Part model, mm, in its own coordinate system. Face numbers are marked on the shaded views. A direction names the side the tool comes from. Round coordinates to 2 decimals unless told otherwise and drop trailing zeros. Write each loop counter-clockwise with the first axis right and the second up, starting at its lowest first coordinate (ties: lowest second). Pieces come first, ordered by that corner, then holes.
1) Saw through at C-C on x = 18.4. Write the cut outline in (y, z), and give its area (3 significant figures).
2) Drill centre lines: L1, parallel to X at y = -27.5, z = 1.15; L2, parallel to X at y = -23.25, z = 3.6; L3, parallel to Y at x = 18.4, z = 3.8. Where is each one in solid material? Low to high.
3) Which spindle directions (+Z, -Z, +X, -X, +Y, -Y) get a long thin tool onto all of the face, cutting with end or side? Do the marked faces 1, 2 and 3. Say none if no direction does.
4) Saw through at B-B on y = -25.75. Write the cut outline in (x, z), and give its area (3 significant figures).
5) Flat gauge pins, fed straight in: pin 1 (6 mm diameter, centred on x = 14.5, y = -29, fed in from -Z); pin 2 (1.5 mm diameter, centred on x = 22, z = 1.5, fed in from +Y). Where does each tip first touch, or does it go through?
6) Saw through at D-D on z = 5.1. Write the cut outline in (x, y), and give its area (3 significant figures).
7) Pull direction Y, two halves, no side cores. Call the marked faces 4, 5 and 6: +Y half, -Y half, draft (parallel to the pull), parting line (faces both ways), or undercut.
8) Saw through at A-A on z = 1.85. Write the cut outline in (x, y), and give its area (3 significant figures).
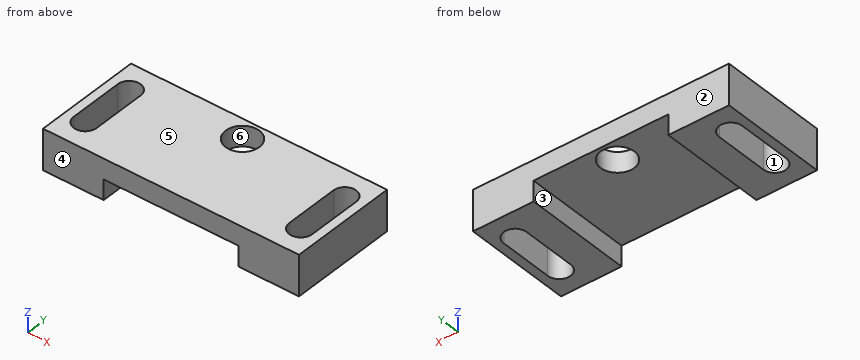
Autodesk Inventor part; units mm, degrees
ref_plane "YZ Plane" through (0, 0, 0) normal (1, 0, 0) x (0, 1, 0)
ref_plane "XZ Plane" through (0, 0, 0) normal (0, 1, 0) x (-1, 0, 0)
ref_plane "XY Plane" through (0, 0, 0) normal (0, 0, 1) x (1, 0, 0)
ref_plane "Work Plane1" through (0, 0, 0) normal (0, 0, 1) x (1, 0, 0)
sketch "Sketch1" plane through (0, 0, 0) normal (0, 0, 1) x (1, 0, 0)
  circle A0 centre (2.4, -23.5737) radius 1.4
  circle A1 centre (34.4, -23.5737) radius 1.4
  line L0 (2.4, -27.5737) -> (2.4, -19.5737) construction
  line L1 (4.1, -27.5737) -> (4.1, -19.5737)
  line L2 (0.7, -19.5737) -> (0.7, -27.5737)
  arc A2 (0.7, -27.5737) -> (4.1, -27.5737) centre (2.4, -27.5737) ccw
  arc A3 (4.1, -19.5737) -> (0.7, -19.5737) centre (2.4, -19.5737) ccw
  line L3 (34.4, -19.5737) -> (34.4, -27.5737) construction
  line L4 (32.7, -19.5737) -> (32.7, -27.5737)
  line L5 (36.1, -27.5737) -> (36.1, -19.5737)
  arc A4 (36.1, -19.5737) -> (32.7, -19.5737) centre (34.4, -19.5737) ccw
  arc A5 (32.7, -27.5737) -> (36.1, -27.5737) centre (34.4, -27.5737) ccw
  line L6 (-0.6, -31.5737) -> (8.4, -31.5737)
  line L7 (8.4, -31.5737) -> (8.4, -15.5737)
  line L8 (8.4, -15.5737) -> (-0.6, -15.5737)
  line L9 (-0.6, -15.5737) -> (-0.6, -31.5737)
  line L10 (37.4, -15.5737) -> (28.4, -15.5737)
  line L11 (28.4, -15.5737) -> (28.4, -31.5737)
  line L12 (28.4, -31.5737) -> (37.4, -31.5737)
  line L13 (37.4, -31.5737) -> (37.4, -15.5737)
  line L14 (8.4, -7.25) -> (8.4, -25.25)
  line L15 (28.4, -7.25) -> (28.4, -25.25)
  point P0 (0, 0)
  dimension "d0" = 4
  dimension "d1" = 3.4
  dimension "d2" = 3.4
  dimension "d3" = 0
  dimension "d4" = 9
  dimension "d5" = 9
  dimension "d6" = 0
  dimension "d7" = 0
  dimension "d8" = 4
  dimension "d9" = 4
extrude "Extrusion1" add sketch "Sketch1" along normal blind 3 contours L9 L8 L7 L6 | L13 L12 L11 L10
sketch "Sketch2" plane through (0, 0, 3) normal (0, 0, 1) x (1, 0, 0)
  line L0 (8.4, -31.5737) -> (8.4, -15.5737)
  line L1 (8.4, -15.5737) -> (-0.6, -15.5737)
  line L2 (-0.6, -15.5737) -> (-0.6, -31.5737)
  line L3 (-0.6, -31.5737) -> (8.4, -31.5737)
  arc A0 (0.7, -27.5737) -> (4.1, -27.5737) centre (2.4, -27.5737) ccw
  line L4 (0.7, -27.5737) -> (0.7, -19.5737)
  arc A1 (4.1, -19.5737) -> (0.7, -19.5737) centre (2.4, -19.5737) ccw
  line L5 (4.1, -19.5737) -> (4.1, -27.5737)
  line L6 (37.4, -15.5737) -> (28.4, -15.5737)
  line L7 (28.4, -15.5737) -> (28.4, -31.5737)
  line L8 (28.4, -31.5737) -> (37.4, -31.5737)
  line L9 (37.4, -31.5737) -> (37.4, -15.5737)
  arc A2 (36.1, -19.5737) -> (32.7, -19.5737) centre (34.4, -19.5737) ccw
  line L10 (36.1, -19.5737) -> (36.1, -27.5737)
  arc A3 (32.7, -27.5737) -> (36.1, -27.5737) centre (34.4, -27.5737) ccw
  line L11 (32.7, -27.5737) -> (32.7, -19.5737)
  line L12 (12.4, 1.5154) -> (12.4, -15.3846)
  line L13 (24.4, 1.5154) -> (24.4, -15.3846)
  circle A4 centre (18.4, -18.5737) radius 2.5
  line L14 (8.4, -15.5737) -> (28.4, -15.5737)
  line L15 (28.4, -31.5737) -> (8.4, -31.5737)
  point P0 (0, 0)
  dimension "d12" = 5
  dimension "d13" = 6
  dimension "d14" = 3
extrude "Extrusion2" add sketch "Sketch2" along normal blind 3
properties part number "10_LED_cylnderlensmount"
Completed:
1. outline: (-31.57, 3) - (-21.07, 3) - (-21.07, 6) - (-31.57, 6) - close; (-16.07, 3) - (-15.57, 3) - (-15.57, 6) - (-16.07, 6) - close
1. area: 33.0 mm2
2. L1: x = -0.6 to 0.7, 4.1 to 8.4, 28.4 to 32.7, 36.1 to 37.4
2. L2: x = -0.6 to 0.7, 4.1 to 32.7, 36.1 to 37.4
2. L3: y = -31.57 to -21.07, -16.07 to -15.57
3. face 1: +Z, -Z
3. face 2: +Z, -Z, +X, -X, +Y
3. face 3: -Z, +Y, -Y
4. outline: (-0.6, 0) - (0.7, 0) - (0.7, 6) - (-0.6, 6) - close; (4.1, 0) - (8.4, 0) - (8.4, 3) - (28.4, 3) - (28.4, 0) - (32.7, 0) - (32.7, 6) - (4.1, 6) - close; (36.1, 0) - (37.4, 0) - (37.4, 6) - (36.1, 6) - close
4. area: 127 mm2
5. pin 1: stops at z = 3
5. pin 2: passes through
6. outline: (-0.6, -31.57) - (37.4, -31.57) - (37.4, -15.57) - (-0.6, -15.57) - close; hole (0.7, -27.57) arc R1.7 ccw to (4.1, -27.57) - (4.1, -19.57) arc R1.7 ccw to (0.7, -19.57) - close; hole circle Ø5 at (18.4, -18.57); hole (32.7, -27.57) arc R1.7 ccw to (36.1, -27.57) - (36.1, -19.57) arc R1.7 ccw to (32.7, -19.57) - close
6. area: 516 mm2
7. face 4: -Y half
7. face 5: draft
7. face 6: undercut
8. outline: (-0.6, -31.57) - (8.4, -31.57) - (8.4, -15.57) - (-0.6, -15.57) - close; (28.4, -31.57) - (37.4, -31.57) - (37.4, -15.57) - (28.4, -15.57) - close; hole (0.7, -27.57) arc R1.7 ccw to (4.1, -27.57) - (4.1, -19.57) arc R1.7 ccw to (0.7, -19.57) - close; hole (32.7, -27.57) arc R1.7 ccw to (36.1, -27.57) - (36.1, -19.57) arc R1.7 ccw to (32.7, -19.57) - close
8. area: 215 mm2
